Autodesk Inventor part; units mm, degrees
ref_plane "YZ Plane" through (0, 0, 0) normal (1, 0, 0) x (0, 1, 0)
ref_plane "XZ Plane" through (0, 0, 0) normal (0, 1, 0) x (-1, 0, 0)
ref_plane "XY Plane" through (0, 0, 0) normal (0, 0, 1) x (1, 0, 0)
sketch "Sketch1" plane through (0, 0, 0) normal (0, 1, 0) x (-1, 0, 0)
  line L0 (21.4313, 42.8625) -> (-21.4313, 42.8625)
  line L1 (-21.4313, 42.8625) -> (-21.4313, -42.8625)
  line L2 (-21.4313, -42.8625) -> (21.4312, -42.8625)
  line L3 (21.4312, -42.8625) -> (21.4313, 42.8625)
  line L4 (0, -60.0075) -> (0, 60.0075) construction
  line L5 (30.0038, 0) -> (-30.0038, 0) construction
  point P0 (0, 0)
  point P1 (0, -42.8625)
  point P2 (-21.4313, 0)
  dimension "d0" = 85.725
  dimension "d1" = 42.8625
extrude "Extrusion1" add sketch "Sketch1" along normal blind 12.7
fillet "Fillet1" radius 4.7625 2 edges at (-21.4312, 12.7, 0) (-21.4312, 0, 0)
fillet "Fillet2" radius 6.35 2 edges at (21.4313, 6.35, 42.8625) (21.4313, 6.35, -42.8625)
properties part number "Onn-USB-Hub"
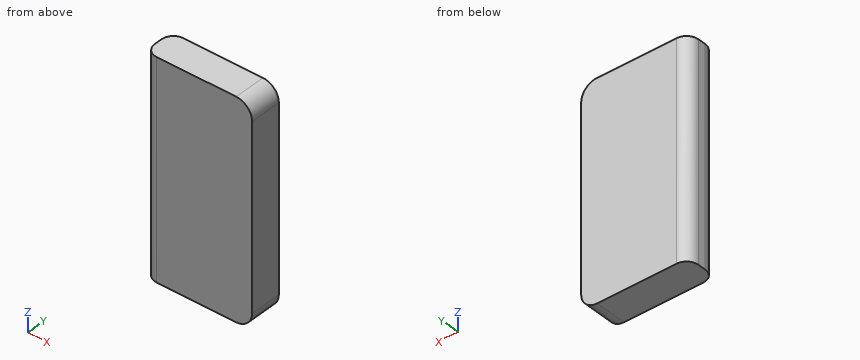
Work out the finished part from the listing and answer in its coordinate system (mm). Give positions to 0.01 mm unless a question says otherwise; leave off trailing zeros. Loops run counter-clockwise (first coordinate to the right, second up) from the corner with the lowest first, then second, coordinate; pieces in that order, holes last. Notation, with made-up numbers: (55.25, -34.5) - (62.25, -34.5) arc R19 ccw to (62.25, 2.5) - close; hole circle Ø9 at (26.25, 0.25). An arc over 180 degrees is marked (long way). Answer in a Markdown table with one row per item. Add a question column.
Q1. The part is cut by section A-A (y = 11.25). Determine the outline of the cut face in (x, z), and give its area (3 significant figures).
Q2. This flat-tipped pin is pushed along its axis until it touches: P1, Ø1.5, axis at y = 3.5, z = 1, coming from the -X side. Where does it stop, or does it pass through?
Q3. Consider line 1 along X through (y, z) = (11.5, 32.5); line 2 along X through (y, z) = (10, -37.5); line 3 along Z through (x, y) = (19.5, 10.5). Determine where each line is inside the solid, lowest interval first.
Solution:
| question | item | result |
|---|---|---|
| 1 | outline | (-20.09, -42.86) - (15.08, -42.86) arc R6.35 ccw to (21.43, -36.51) - (21.43, 36.51) arc R6.35 ccw to (15.08, 42.86) - (-20.09, 42.86) - close |
| 1 | area | 3,540 mm² |
| 2 | P1 | stops at x = -21.4 |
| 3 | line 1 | x = -19.83 to 21.43 |
| 3 | line 2 | x = -20.96 to 21.35 |
| 3 | line 3 | z = -41.07 to 41.07 |
